Autodesk Inventor part; units mm, degrees
ref_plane "Work Plane1" through (0, 75, 0) normal (0, 1, 0) x (-1, 0, 0)
ref_plane "YZ Plane" through (0, 0, 0) normal (1, 0, 0) x (0, 1, 0)
ref_plane "XY Plane" through (0, 0, 0) normal (0, 0, 1) x (1, 0, 0)
sketch "Sketch1" plane through (0, 0, 0) normal (0, 0, 1) x (1, 0, 0)
  circle A0 centre (0, 0) radius 54.5
  circle A1 centre (0, 0) radius 75
  circle A2 centre (0, 0) radius 56.5
  circle A3 centre (0, 0) radius 62.5
  circle A4 centre (0, 0) radius 69
  line L0 (0, 0) -> (0, 69) construction
  line L1 (0, 0) -> (26.4052, 63.7477) construction
  line L2 (0, 0) -> (69, 0) construction
  circle A5 centre (26.4052, 63.7477) radius 4
  dimension "d0" = 109
  dimension "d1" = 150
  dimension "d2" = 113
  dimension "d3" = 125
  dimension "d4" = 138
  dimension "d16" = 67.5
  dimension "d17" = 8
extrude "Extrusion1" add sketch "Sketch1" along normal blind 20 contours A2
extrude "Extrusion2" add sketch "Sketch1" along normal blind 15 contours A3
extrude "Extrusion3" add sketch "Sketch1" along normal blind 20 contours A1 | A4 A5 | A5 A4 | A4 A5
ref_plane "Work Plane1" through (0, 75, 0) normal (0, 1, 0) x (-1, 0, 0)
sketch "Sketch2" plane through (0, 75, 0) normal (0, 1, 0) x (-1, 0, 0)
  line L0 (0, 0) -> (0, 10) construction
  circle A0 centre (0, 10) radius 6.858
  dimension "d12" = 10
  dimension "d13" = 13.716
extrude "Extrusion4" cut sketch "Sketch2" against normal blind 18
extrude "Extrusion5" cut sketch "Sketch1" along normal through all contours A5 A4 | A4 A5 picked at (25.7495, 62.5769) picked at (26.9375, 64.9608)
thread "Thread2"
pattern_circular "Circular Pattern2" count 8 over 360 about axis through (0, 0, -10) along (0, 0, 1) of "Extrusion5"
thread "Thread13"
thread "Thread14"
thread "Thread15"
thread "Thread16"
thread "Thread17"
thread "Thread18"
thread "Thread19"
thread "Thread20"
thread "Thread21"
properties part number "front" material "Aluminum 6061"
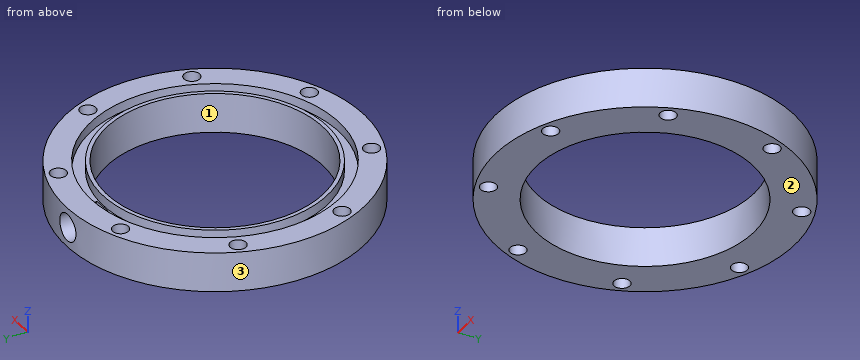
Geometry: final body of the model. Coordinates: model frame, mm. Face numbers are marked on the shaded views. Give positions to 0.01 mm unless a question says otherwise; leave off trailing zeros. Write each loop counter-clockwise with the first axis right and the second up, starting at its lowest first coordinate (ties: lowest second). Pieces come first, ordered by that corner, then holes. Notation, with made-up numbers: M -34,32 L -23,32 A15 ccw -23,51 Z; hole C -13.5,20.5 d6. An arc over 180 degrees is marked long. Answer in a Markdown table with one row per item. Add a question column.
(1) Section B-B on x = 0. Return loops of the section in (y, z).
(2) Section D-D on y = 28.5. Return loops of the section in (x, z).
(3) Section A-A on y = 0. Return loops of the section in (x, z), and give its area (3 significant figures).
(4) Section C-C on x = -43. Return loops of the section in (y, z), and give its area (3 significant figures).
(5) First-contact query: pin 1 (1 mm diameter, centred on y = -50, z = 16, fed in from +X); pin 2 (2 mm diameter, centred on y = 39, z = 2.5, fed in from +X); pin 3 (8 mm diameter, centred on x = -2.5, z = 7.5, fed in from +Y); pin 4 (13 mm diameter, centred on x = 63.75, y = -26.41, fed in from +Z). Flat tips, straight axial feed; report the tip coordinate or a pass-through.
(6) Mould query, pull axis Y, two halves, no side actions, for the marked faces 1, 2 and 3. Classes: +Y half, -Y half, draft (parallel to the pull), parting line (faces both ways), or undercut.
(7) Ray query, line 1 (Y direction, x = 34.5, z = 18.5); line 2 (Y direction, x = 23.5, z = 10.75); line 3 (X direction, y = -8, z = 17.5). Return the intervals inside material, ascending.
Result set:
| question | item | result |
|---|---|---|
| 1 | outline | M -75,0 L -54.5,0 L -54.5,20 L -56.5,20 L -56.5,15 L -62.5,15 L -62.5,20 L -75,20 Z; M 54.5,0 L 75,0 L 75,3.14 L 57,3.14 L 57,15 L 56.5,15 L 56.5,20 L 54.5,20 Z; M 62.5,16.86 L 75,16.86 L 75,20 L 62.5,20 Z |
| 2 | outline | M -69.37,0 L -67.16,0 L -67.16,20 L -69.37,20 Z; M -60.34,0 L -46.45,0 L -46.45,20 L -48.79,20 L -48.79,15 L -55.62,15 L -55.62,20 L -60.34,20 Z; M 46.45,0 L 60.34,0 L 60.34,20 L 55.62,20 L 55.62,15 L 48.79,15 L 48.79,20 L 46.45,20 Z; M 67.16,0 L 69.37,0 L 69.37,20 L 67.16,20 Z |
| 3 | outline | M -75,0 L -54.5,0 L -54.5,20 L -56.5,20 L -56.5,15 L -62.5,15 L -62.5,20 L -75,20 Z; M 54.5,0 L 75,0 L 75,20 L 62.5,20 L 62.5,15 L 56.5,15 L 56.5,20 L 54.5,20 Z |
| 3 | area | 760 mm^2 |
| 4 | outline | M -61.45,0 L -33.49,0 L -33.49,20 L -36.65,20 L -36.65,15 L -45.36,15 L -45.36,20 L -61.45,20 Z; M 33.49,0 L 61.45,0 L 61.45,20 L 45.36,20 L 45.36,15 L 36.65,15 L 36.65,20 L 33.49,20 Z |
| 4 | area | 1,030 mm^2 |
| 5 | pin 1 | stops at x = 56.34 |
| 5 | pin 2 | stops at x = 64.66 |
| 5 | pin 3 | stops at y = 74.97 |
| 5 | pin 4 | stops at z = 20 |
| 6 | face 1 | undercut |
| 6 | face 2 | draft |
| 6 | face 3 | parting line |
| 7 | line 1 | y = -66.59 to -52.12, -44.74 to -42.19, 42.19 to 44.74, 52.12 to 66.59 |
| 7 | line 2 | y = -71.22 to -66.5, -61 to -49.17, 49.17 to 61, 66.5 to 71.22 |
| 7 | line 3 | x = -74.57 to -61.99, -55.93 to -53.91, 53.91 to 55.93, 61.99 to 74.57 |
